Check sheet for the modelled part. Datum: model origin and axes. Units: mm. A direction names the side the tool comes from. Coordinates: 2 decimals unless noted, no trailing zeros. Loops run counter-clockwise (first coordinate to the right, second up) from the corner with the lowest first, then second, coordinate; pieces in that order, holes last. Notation, with made-up numbers: (-9.75, 71.25) - (3.25, 71.25) arc R22 ccw to (3.25, 77.25) - close; hole circle Ø11 at (48.5, -9). An arc over 180 degrees is marked (long way). Write each question's results on one line, items separated by ' | '. Start each with the question number.
1. Thickness scan on line 1 (Y direction, x = 37, z = -51.5); line 2 (Y direction, x = 25, z = -23); line 3 (Z direction, x = 14, y = 22.5). Record the ranges inside material, lowest first. Write a range as [from, to].
2. Cross-section at D-D (z = -26). Record the cut outline in (x, y), and give its area (3 significant figures).
3. Draft check along Y on faces 1 (the face through (35, 4.911, -34)), 2 (the face through (38, 1, -38)), 3 (the face through (35, 3, -34)), 4 (the face through (35, 66.802, -34)). Enter one of: released by +Y, released by -Y, zero draft, split by the parting line, or undercut.
4. Cross-section at A-A (z = -58.5). Record the cut outline in (x, y).
5. Cross-section at C-C (x = 41). Record the cut outline in (y, z), and give its area (3 significant figures).
6. Tool access check on faces 5 (the face through (50.7, 34.7, -59.56)), 6 (the face through (10.29, 34.7, -19.15)), 7 (the face through (25.66, 35.15, -43.62)). Record the directions out of +Z, -Z, +X, -X, +Y, -Y that give a thin tool (end or side, any length) a straight path to the whole face; none if there is none.
7. Gauge pin test, flat ends, axial feed: P1, Ø1, axis at x = 20.5, z = -55.5, coming from the -Y side; P2, Ø10, axis at y = 33.5, z = -34.5, coming from the +X side; P3, Ø3, axis at x = 62, y = 62, coming from the +Z side. Record the tip position at first contact, or that the pin passes through.
8. Cross-section at B-B (y = 18). Record the cut outline in (x, z), and give its area (3 significant figures).
```python
from build123d import *

# Parameters (mm, degrees)
SKETCH1_W           = 69.85
SKETCH1_H           = 69.85
BOSS_EXTRUDE1_DEPTH = 69.85
CUT_EXTRUDE2_DEPTH  = 100
SKETCH3_W           = 92.734817332
SKETCH3_H           = 63.802
SKETCH3_W_2         = 88.628817955
SKETCH3_H_2         = 59.858884928
BOSS_EXTRUDE2_DEPTH = 2.032
SKETCH4_W           = 57.15
SKETCH4_H           = 31.75
CUT_EXTRUDE3_DEPTH  = 12.7


with BuildPart() as part:
    # Sketch1 → Boss-Extrude1 (new body)
    with BuildSketch(Plane(origin=(0, 0, 0), x_dir=(1, 0, 0), z_dir=(0, 1, 0))):
        with Locations((34.925, 34.925)):
            Rectangle(SKETCH1_W, SKETCH1_H)
    extrude(amount=BOSS_EXTRUDE1_DEPTH)

    # Sketch2 → Cut-Extrude2 (cut)
    with BuildSketch(Plane(origin=(0, 0, 0), x_dir=(0.707106781, 0, -0.707106781), z_dir=(0.707106781, 0, 0.707106781))):
        Polygon((98.782817332, 69.85), (98.782817332, 0), (49.391408666, 0), (0, 0), (0, 69.85), (49.391408666, 69.85), align=None)
    extrude(amount=CUT_EXTRUDE2_DEPTH, mode=Mode.SUBTRACT)

    # Sketch3 → Boss-Extrude2 (add)
    with BuildSketch(Plane(origin=(0, 0, 0), x_dir=(0.707106781, 0, -0.707106781), z_dir=(0.707106781, 0, 0.707106781))):
        with Locations((49.367408666, 34.901)):
            Rectangle(SKETCH3_W, SKETCH3_H)
        with Locations((49.388408355, 34.840557536)):
            Rectangle(SKETCH3_W_2, SKETCH3_H_2, mode=Mode.SUBTRACT)
    extrude(amount=BOSS_EXTRUDE2_DEPTH)

    # Sketch4 → Cut-Extrude3 (cut)
    with BuildSketch(Plane(origin=(0, 0, 0), x_dir=(0.707106781, 0, -0.707106781), z_dir=(0.707106781, 0, 0.707106781))):
        with Locations((49.391408666, 34.925)):
            Rectangle(SKETCH4_W, SKETCH4_H)
    extrude(amount=-CUT_EXTRUDE3_DEPTH, mode=Mode.SUBTRACT)


solid = part.part
```
Established:
1) line 1: [0, 19.05], [50.8, 69.85] | line 2: [3, 4.91], [64.77, 66.8] | line 3: [-69.85, -31.96], [-15.44, -14]
2) outline: (0, 0) - (26, 0) - (26, 3) - (28.87, 3) - (28.87, 4.91) - (26, 4.91) - (26, 19.05) - (8.04, 19.05) - (8.04, 50.8) - (26, 50.8) - (26, 64.77) - (28.87, 64.77) - (28.87, 66.8) - (26, 66.8) - (26, 69.85) - (0, 69.85) - close | area: 1,260 mm^2
3) face 1: undercut | face 2: zero draft | face 3: released by -Y | face 4: released by +Y
4) outline: (0, 0) - (58.5, 0) - (58.5, 3) - (61.37, 3) - (61.37, 4.91) - (58.5, 4.91) - (58.5, 64.77) - (61.37, 64.77) - (61.37, 66.8) - (58.5, 66.8) - (58.5, 69.85) - (0, 69.85) - close; hole (40.54, 19.05) - (51.76, 19.05) - (51.76, 50.8) - (40.54, 50.8) - close
5) outline: (0, -69.85) - (69.85, -69.85) - (69.85, -41) - (66.8, -41) - (66.8, -38.13) - (64.77, -38.13) - (64.77, -41) - (50.8, -41) - (50.8, -58.96) - (19.05, -58.96) - (19.05, -41) - (4.91, -41) - (4.91, -38.13) - (3, -38.13) - (3, -41) - (0, -41) - close | area: 1,460 mm^2
6) face 5: +Z | face 6: +X | face 7: none
7) P1: y = 0 | P2: x = 21.54 | P3: z = -60.5
8) outline: (0, -69.85) - (69.85, -69.85) - (67.69, -67.69) - (69.13, -66.26) - (67.69, -64.82) - (66.26, -66.26) - (3.59, -3.59) - (5.02, -2.15) - (3.56, -0.68) - (2.12, -2.12) - (0, 0) - close | area: 2,450 mm^2
